For this review, take the finished solid that the model builds, in its own axes (mm). A direction names the side the tool comes from. Give positions to 0.01 mm unless a question says otherwise; leave off trailing zeros. Loops run counter-clockwise (first coordinate to the right, second up) from the corner with the lowest first, then second, coordinate; pieces in that order, holes last.
Autodesk Inventor part; units mm, degrees
ref_plane "YZ Plane" through (0, 0, 0) normal (1, 0, 0) x (0, 1, 0)
ref_plane "XZ Plane" through (0, 0, 0) normal (0, 1, 0) x (-1, 0, 0)
ref_plane "XY Plane" through (0, 0, 0) normal (0, 0, 1) x (1, 0, 0)
sketch "Sketch1" plane through (0, 0, 0) normal (0, 0, 1) x (1, 0, 0)
  line L0 (-30, 70) -> (30, 70)
  line L1 (30, 70) -> (30, -70)
  line L2 (30, -70) -> (-30, -70)
  line L3 (-30, -70) -> (-30, 70)
  point P0 (0, 0)
  dimension "d0" = 60
  dimension "d1" = 140
  dimension "d2" = 30
  dimension "d3" = 70
extrude "Extrusion1" add sketch "Sketch1" along normal blind 3.4163
sketch "Sketch2" plane through (0, 0, 3.4163) normal (0, 0, 1) x (1, 0, 0)
  line L0 (-30, 70) -> (-30, -70)
  line L1 (-30, -70) -> (30, -70)
  circle A0 centre (-20, -60) radius 2.625
  point P0 (0, 0)
  dimension "d6" = 5.25
  dimension "d7" = 10
  dimension "d8" = 10
extrude "Extrusion2" cut sketch "Sketch2" against normal through all
pattern_linear "Rectangular Pattern1" count 2 spacing 40 along (1, 0, 0) count 2 spacing 20 along (0, 1, 0) of "Extrusion2"
sketch "Sketch3" plane through (0, 0, 3.4163) normal (0, 0, 1) x (1, 0, 0)
  line L0 (-30, 70) -> (-30, -70)
  line L1 (-30, -70) -> (30, -70)
  arc A0 (-22.625, -5) -> (-17.375, -5) centre (-20, -5) ccw
  arc A1 (-17.375, 20) -> (-22.625, 20) centre (-20, 20) ccw
  line L2 (-22.625, 20) -> (-22.625, -5)
  line L3 (-17.375, -5) -> (-17.375, 20)
  point P0 (0, 0)
  dimension "d17" = 5.25
  dimension "d18" = 65
  dimension "d19" = 10
  dimension "d20" = 5.25
  dimension "d22" = 10
  dimension "d26" = 25
  dimension "d27" = 25
extrude "Extrusion3" cut sketch "Sketch3" against normal through all
sketch "Sketch4" plane through (0, 0, 3.4163) normal (0, 0, 1) x (1, 0, 0)
  line L0 (-30, 70) -> (-30, -70)
  line L1 (-30, -70) -> (30, -70)
  line L2 (-6.5, 32) -> (7.5, 32)
  line L3 (7.5, 32) -> (7.5, 29)
  line L4 (7.5, 29) -> (-6.5, 29)
  line L5 (-6.5, 29) -> (-6.5, 32)
  point P0 (0, 0)
  dimension "d28" = 14
  dimension "d29" = 3
  dimension "d30" = 99
  dimension "d31" = 23.5
extrude "Extrusion4" cut sketch "Sketch4" against normal through all
sketch "Sketch5" plane through (0, 0, 3.4163) normal (0, 0, 1) x (1, 0, 0)
  line L0 (30, 70) -> (-30, 70)
  line L1 (-30, 70) -> (-30, -70)
  line L2 (-30, -70) -> (30, -70)
  circle A0 centre (0, 46) radius 2.625
  arc A1 (-20.625, 62.625) -> (-20.625, 57.375) centre (-20.625, 60) ccw
  arc A2 (15.625, 62.625) -> (15.625, 57.375) centre (15.625, 60) ccw
  arc A3 (-15.375, 57.375) -> (-15.375, 62.625) centre (-15.375, 60) ccw
  line L3 (-20.625, 62.625) -> (-15.375, 62.625)
  line L4 (-15.375, 57.375) -> (-20.625, 57.375)
  arc A4 (20.875, 57.375) -> (20.875, 62.625) centre (20.875, 60) ccw
  line L5 (20.875, 62.625) -> (15.625, 62.625)
  line L6 (15.625, 57.375) -> (20.875, 57.375)
  point P0 (0, 0)
  dimension "d34" = 5.25
  dimension "d35" = 116
  dimension "d36" = 5.25
  dimension "d37" = 5.25
  dimension "d38" = 10
  dimension "d39" = 10
  dimension "d40" = 36.25
  dimension "d41" = 9.375
  dimension "d48" = 5.25
  dimension "d49" = 5.25
  dimension "d50" = 10
  dimension "d51" = 5.25
  dimension "d52" = 5.25
  dimension "d53" = 5.25
  dimension "d54" = 10
  dimension "d55" = 5.25
extrude "Extrusion5" cut sketch "Sketch5" against normal blind 3.4163
pattern_linear "Rectangular Pattern2" count 3 spacing 20 along (1, 0, 0) of "Extrusion3"
fillet "Fillet1" radius 5 4 edges at (-30, 70, 1.7082) (30, 70, 1.7082) (30, -70, 1.7082) (-30, -70, 1.7082)
equation "\"d20\" = d17"
equation "\"d39\" = d38"
properties part number "26028-01" material "Steel, Mild"
Item 1: Take a section at A-A on y = 60. Give the boundary of the cut face in (x, z).
Answer:
outline: (-30, 0) - (-23.25, 0) - (-23.25, 3.42) - (-30, 3.42) - close; (-12.75, 0) - (13, 0) - (13, 3.42) - (-12.75, 3.42) - close; (23.5, 0) - (30, 0) - (30, 3.42) - (23.5, 3.42) - close
Item 2: Take a section at B-B on x = 0. Give the boundary of the cut face in (y, z) (3 decimals), and give its area (3 significant figures).
Answer:
outline: (-70, 0) - (-7.625, 0) - (-7.625, 3.416) - (-70, 3.416) - close; (22.625, 0) - (29, 0) - (29, 3.416) - (22.625, 3.416) - close; (32, 0) - (43.375, 0) - (43.375, 3.416) - (32, 3.416) - close; (48.625, 0) - (70, 0) - (70, 3.416) - (48.625, 3.416) - close
area: 347 mm2
Item 3: For L1, parallel to Y at x = 20, z = 2.65 (3 decimals); L2, parallel to X at y = 15.5, z = 2.2 (3 decimals); L3, parallel to X at y = 21.5, z = 0.4, list the stretches that pass through material, from the lowest coordinate up.
Answer:
L1: y = -70 to -62.625, -57.375 to -42.625, -37.375 to -7.625, 22.625 to 57.375, 62.625 to 70
L2: x = -30 to -22.625, -17.375 to -2.625, 2.625 to 17.375, 22.625 to 30
L3: x = -30 to -22.15, -17.85 to -2.15, 2.15 to 17.85, 22.15 to 30
Item 4: Take a section at C-C on y = -40. Give the boundary of the cut face in (x, z) (3 decimals).
Answer:
outline: (-30, 0) - (-22.625, 0) - (-22.625, 3.416) - (-30, 3.416) - close; (-17.375, 0) - (17.375, 0) - (17.375, 3.416) - (-17.375, 3.416) - close; (22.625, 0) - (30, 0) - (30, 3.416) - (22.625, 3.416) - close
Item 5: The part is to be moulded in two halves that separate along Y. For faces 3 (the cylindrical face through (-20.342, -57.397, 1.732)), 4 (the cylindrical face through (-28, 69, 2)), 5 (the cylindrical face through (28, -69, 2)), say which applies: released by +Y, released by -Y, zero draft, split by the parting line, or undercut.
Answer:
face 3: undercut
face 4: released by +Y
face 5: released by -Y
Item 6: Take a section at D-D on z = 2.45. State how many separate pieces and enclosed holes the cut face has, and give its area (3 significant figures).
Answer:
separate pieces: 1
enclosed holes: 11
area: 7,670 mm2
Item 7: Tool access review of faces 1 (the flat face through (0, -70, 2)), 2 (the cylindrical face through (20.058, 22.624, 1.732)): name each direction out of +Z, -Z, +X, -X, +Y, -Y from which nothing blocks a thin tool from reaching the whole face with its end or side.
Answer:
face 1: +Z, -Z, +X, -X, -Y
face 2: +Z, -Z
